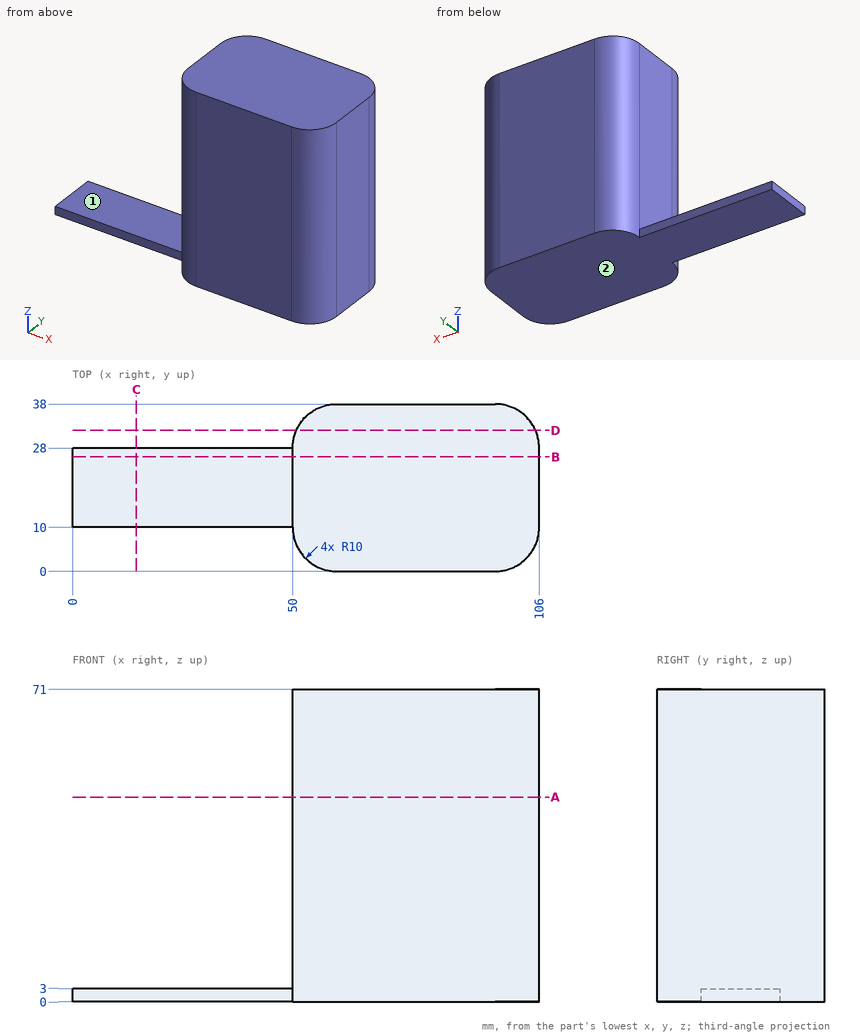
Geometry: see drawing. Coordinates: mm, zero at the bounding-box minimum. A direction names the side the tool comes from. Round coordinates to 2 decimals unless told otherwise and drop trailing zeros. Write each loop counter-clockwise with the first axis right and the second up, starting at its lowest first coordinate (ties: lowest second). Pieces come first, ordered by that corner, then holes.
1) Cut plane C-C (x = 14.5). Return the cut outline in (y, z), then the cut area to 3 significant figures.
2) Cut plane B-B (y = 26). Return the cut outline in (x, z), then the cut area to 3 significant figures.
3) Cut plane D-D (y = 32). Return the cut outline in (x, z), then the cut area to 3 significant figures.
4) Ray query, L1, parallel to X at y = 20, z = 53.5; L2, parallel to Z at x = 26, y = 24; L3, parallel to X at y = 8, z = 32. Return the intervals inside material, ascending.
5) Reachability of the marked faces 1 and 2 from +Z, -Z, +X, -X, +Y, -Y: full face, straight path, thin tool, end or side. Return the list, or none.
6) Contact query for flat-ended pins moving along their axis: P1, Ø2.5, axis at x = 18.5, z = 1, coming from the +Y side; P2, Ø1.5, axis at x = 28, z = 1.5, coming from the -Y side; P3, Ø14.5, axis at y = 23, z = 39, coming from the -X side. Output: stop coordinate, or through.
7) Cut plane A-A (z = 46.5). Return the cut outline in (x, y), then the cut area to 3 significant figures.
Geometry says:
1. outline: (10, 0) - (28, 0) - (28, 3) - (10, 3) - close
1. area: 54.0 mm2
2. outline: (0, 0) - (106, 0) - (106, 71) - (50, 71) - (50, 3) - (0, 3) - close
2. area: 4,130 mm2
3. outline: (50.83, 0) - (105.17, 0) - (105.17, 71) - (50.83, 71) - close
3. area: 3,860 mm2
4. L1: x = 50 to 106
4. L2: z = 0 to 3
4. L3: x = 50.2 to 105.8
5. face 1: +Z, -X, +Y, -Y
5. face 2: -Z, +X, -X, +Y, -Y
6. P1: stops at y = 28
6. P2: stops at y = 10
6. P3: stops at x = 50
7. outline: (50, 10) arc R10 ccw to (60, 0) - (96, 0) arc R10 ccw to (106, 10) - (106, 28) arc R10 ccw to (96, 38) - (60, 38) arc R10 ccw to (50, 28) - close
7. area: 2,040 mm2
